```python
from build123d import *

# Parameters (mm, degrees)
SKETCH006_W     = 112.91
SKETCH006_H     = 87.54
SKETCH006_R     = 3
SKETCH006_R_2   = 2.65
SKETCH006_R_3   = 36
PAD005_DEPTH    = 1.6
CHAMFER_SIZE    = 1
SKETCH007_W     = 112.91
SKETCH007_H     = 87.54
SKETCH007_R     = 3
PAD006_DEPTH    = 1.8
SKETCH009_W     = 112.91
SKETCH009_H     = 87.54
SKETCH009_R     = 1.75
PAD007_DEPTH    = 28.2
SKETCH008_W     = 44
SKETCH008_H     = 25
POCKET_DEPTH    = 1.22
POCKET001_DEPTH = 1.22
SKETCH011_W     = 95.03
SKETCH011_H     = 22
POCKET002_DEPTH = 1.22
SKETCH012_W     = 42.2
SKETCH012_H     = 22
SKETCH012_W_2   = 15.44
SKETCH012_H_2   = 2
SKETCH012_W_3   = 12.5
SKETCH012_H_3   = 12
POCKET003_DEPTH = 1.22
FILLET001_R     = 1


with BuildPart() as part:
    # Sketch006 → Pad005 (new body)
    with BuildSketch(Plane.XY):
        Rectangle(SKETCH006_W, SKETCH006_H)
        with Locations((-50.925, 38.05)):
            Circle(SKETCH006_R, mode=Mode.SUBTRACT)
        with Locations((50.925, 38.05)):
            Circle(SKETCH006_R, mode=Mode.SUBTRACT)
        with Locations((-50.925, -38.05)):
            Circle(SKETCH006_R, mode=Mode.SUBTRACT)
        with Locations((50.925, -38.05)):
            Circle(SKETCH006_R, mode=Mode.SUBTRACT)
        with Locations((-43.265, 35.75)):
            Circle(SKETCH006_R_2, mode=Mode.SUBTRACT)
        with Locations((28.235, 35.75)):
            Circle(SKETCH006_R_2, mode=Mode.SUBTRACT)
        with Locations((28.235, -35.75)):
            Circle(SKETCH006_R_2, mode=Mode.SUBTRACT)
        with Locations((-43.265, -35.75)):
            Circle(SKETCH006_R_2, mode=Mode.SUBTRACT)
        with Locations((-7.515, 0)):
            Circle(SKETCH006_R_3, mode=Mode.SUBTRACT)
    extrude(amount=PAD005_DEPTH)

    # Chamfer
    chamfer_edges = [part.edges().sort_by_distance(p)[0] for p in [
        (-45.915, 35.75, 1.6),
        (25.585, 35.75, 1.6),
        (-45.915, -35.75, 1.6),
        (25.585, -35.75, 1.6),
    ]]
    chamfer(chamfer_edges, length=CHAMFER_SIZE)

    # Sketch007 → Pad006 (join)
    with BuildSketch(Plane.XY.offset(1.6)):
        Rectangle(SKETCH007_W, SKETCH007_H)
        with Locations((-50.925, 38.05)):
            Circle(SKETCH007_R, mode=Mode.SUBTRACT)
        with Locations((50.925, 38.05)):
            Circle(SKETCH007_R, mode=Mode.SUBTRACT)
        with Locations((-50.925, -38.05)):
            Circle(SKETCH007_R, mode=Mode.SUBTRACT)
        with Locations((50.925, -38.05)):
            Circle(SKETCH007_R, mode=Mode.SUBTRACT)
        with BuildLine():
            Line((-47.515, 42.55), (47.515, 42.55))
            Line((47.515, 42.55), (47.515, 38.05))
            ThreePointArc((47.515, 38.05), (48.513766, 35.638766), (50.925, 34.64))
            Line((55.235, 34.64), (50.925, 34.64))
            Line((55.235, -34.64), (55.235, 34.64))
            Line((55.235, -34.64), (50.925, -34.64))
            ThreePointArc((50.925, -34.64), (48.513766, -35.638766), (47.515, -38.05))
            Line((47.515, -42.55), (47.515, -38.05))
            Line((-47.515, -42.55), (47.515, -42.55))
            Line((-47.515, -42.55), (-47.515, -38.05))
            ThreePointArc((-47.515, -38.05), (-48.513766, -35.638766), (-50.925, -34.64))
            Line((-55.235, -34.64), (-50.925, -34.64))
            Line((-55.235, 34.64), (-55.235, -34.64))
            Line((-55.235, 34.64), (-50.925, 34.64))
            ThreePointArc((-50.925, 34.64), (-48.513766, 35.638766), (-47.515, 38.05))
            Line((-47.515, 42.55), (-47.515, 38.05))
        make_face(mode=Mode.SUBTRACT)
    extrude(amount=PAD006_DEPTH)

    # Sketch009 → Pad007 (join)
    with BuildSketch(Plane.XY.offset(3.4)):
        Rectangle(SKETCH009_W, SKETCH009_H)
        with Locations((-50.925, 38.05)):
            Circle(SKETCH009_R, mode=Mode.SUBTRACT)
        with Locations((50.925, 38.05)):
            Circle(SKETCH009_R, mode=Mode.SUBTRACT)
        with Locations((-50.925, -38.05)):
            Circle(SKETCH009_R, mode=Mode.SUBTRACT)
        with Locations((50.925, -38.05)):
            Circle(SKETCH009_R, mode=Mode.SUBTRACT)
        with BuildLine():
            Line((-47.515, 42.55), (47.515, 42.55))
            Line((47.515, 42.55), (47.515, 38.05))
            ThreePointArc((47.515, 38.05), (48.513766, 35.638766), (50.925, 34.64))
            Line((55.235, 34.64), (50.925, 34.64))
            Line((55.235, -34.64), (55.235, 34.64))
            Line((55.235, -34.64), (50.925, -34.64))
            ThreePointArc((50.925, -34.64), (48.513766, -35.638766), (47.515, -38.05))
            Line((47.515, -42.55), (47.515, -38.05))
            Line((-47.515, -42.55), (47.515, -42.55))
            Line((-47.515, -42.55), (-47.515, -38.05))
            ThreePointArc((-47.515, -38.05), (-48.513766, -35.638766), (-50.925, -34.64))
            Line((-55.235, -34.64), (-50.925, -34.64))
            Line((-55.235, 34.64), (-55.235, -34.64))
            Line((-55.235, 34.64), (-50.925, 34.64))
            ThreePointArc((-50.925, 34.64), (-48.513766, 35.638766), (-47.515, 38.05))
            Line((-47.515, 42.55), (-47.515, 38.05))
        make_face(mode=Mode.SUBTRACT)
    extrude(amount=PAD007_DEPTH)

    # Sketch008 → Pocket (cut)
    with BuildSketch(Plane(origin=(56.455, 0, 1.6), x_dir=(0, 1, 0), z_dir=(1, 0, 0))):
        with Locations((1.85, 17.5)):
            Rectangle(SKETCH008_W, SKETCH008_H)
    extrude(amount=-POCKET_DEPTH, mode=Mode.SUBTRACT)

    # Sketch010 → Pocket001 (cut)
    with BuildSketch(Plane(origin=(-56.455, 0, 1.6), x_dir=(0, -1, 0), z_dir=(-1, 0, 0))):
        Polygon((-34.65, 30), (18.85, 30), (18.85, 12), (10.85, 12), (10.85, 20), (-34.65, 20), align=None)
    extrude(amount=-POCKET001_DEPTH, mode=Mode.SUBTRACT)

    # Sketch011 → Pocket002 (cut)
    with BuildSketch(Plane(origin=(0, -43.77, 1.6), x_dir=(1, 0, 0), z_dir=(0, -1, 0))):
        with Locations((0, 19)):
            Rectangle(SKETCH011_W, SKETCH011_H)
    extrude(amount=-POCKET002_DEPTH, mode=Mode.SUBTRACT)

    # Sketch012 → Pocket003 (cut)
    with BuildSketch(Plane(origin=(0, 43.77, 1.6), x_dir=(-1, 0, 0), z_dir=(0, 1, 0))):
        with Locations((-25.735, 19)):
            Rectangle(SKETCH012_W, SKETCH012_H)
        with Locations((4.855, 29)):
            Rectangle(SKETCH012_W_2, SKETCH012_H_2)
        with Locations((24.785, 24)):
            Rectangle(SKETCH012_W_3, SKETCH012_H_3)
    extrude(amount=-POCKET003_DEPTH, mode=Mode.SUBTRACT)

    # Fillet001
    fillet001_edges = [part.edges().sort_by_distance(p)[0] for p in [
        (56.455, -43.77, 15.8),
        (56.455, 0, 0),
        (0, -43.77, 0),
        (56.455, 43.77, 15.8),
        (0, 43.77, 0),
        (-56.455, 0, 0),
        (-56.455, -43.77, 15.8),
        (-56.455, 43.77, 15.8),
        (-48.513766, -35.638766, 1.6),
        (-55.235, 0, 1.6),
        (0, -42.55, 1.6),
        (-48.513766, 35.638766, 1.6),
        (48.513766, -35.638766, 1.6),
        (0, 42.55, 1.6),
        (48.513766, 35.638766, 1.6),
        (55.235, 0, 1.6),
    ]]
    fillet(fillet001_edges, radius=FILLET001_R)


solid = part.part
```
Model file for the job. Use its own axes, mm. A direction names the side the tool comes from. Round coordinates to 2 decimals unless told otherwise and drop trailing zeros. Order: outer loops, then holes, each group sorted by start corner. A loop starts at its lowest first (then second) coordinate and runs counter-clockwise, first axis right, second up. Notation, with made-up numbers: M -23,-25.5 L 24,-25.5 A19 ccw 24,-10.5 Z; hole C 70,73 d10. An arc over 180 degrees is marked long. Use CSV: the item, a comma, the result in double quotes.
Item 1: Which spindle directions (+Z, -Z, +X, -X, +Y, -Y) get a long thin tool onto all of the face, cutting with end or side? Do faces 4 (the face through (53, 34.64, 17)), 5 (the face through (-49, 38, 3.4)), 6 (the face through (49.635, 39.233, 17.303)). Say none if no direction does.
Worked answers:
face 4,"+Z"
face 5,"-Z"
face 6,"+Z, -Z"
Item 2: Saw through at D-D (x = -16.5). List the corners of the cut face in (y, z).
Worked answers:
outline,"M -43.77,1 A1 ccw -42.77,0 L -34.86,0 L -34.86,1.6 L -41.55,1.6 A1 cw -42.55,2.6 L -42.55,9.6 L -43.77,9.6 Z; M 34.86,0 L 42.77,0 A1 ccw 43.77,1 L 43.77,31.6 L 42.55,31.6 L 42.55,2.6 A1 cw 41.55,1.6 L 34.86,1.6 Z"
Item 3: Saw through at C-C (z = 17). State how many separate pieces and enclosed holes the cut face has, plus the area to 3 significant figures.
Worked answers:
separate pieces,"4"
enclosed holes,"4"
area,"447 mm²"
Item 4: Saw through at A-A (y = 0). List the corners of the cut face in (x, z) (3 decimals), plus the area to 3 significant figures.
Worked answers:
outline,"M -56.455,1 A1 ccw -55.455,0 L -43.515,0 L -43.515,1.6 L -54.235,1.6 A1 cw -55.235,2.6 L -55.235,21.6 L -56.455,21.6 Z; M 28.485,0 L 55.455,0 A1 ccw 56.455,1 L 56.455,6.6 L 55.235,6.6 L 55.235,2.6 A1 cw 54.235,1.6 L 28.485,1.6 Z"
area,"96.0 mm²"
Item 5: Probe probe 1 along X at (y, z) = (38, 23) (3 decimals); probe 2 along Y at (x, z) = (-1, 3); probe 3 along X at (y, z) = (32, 5.5) (3 decimals). List the from-to ranges inside material, lowest first.
Worked answers:
probe 1,"-56.455 to -52.674, -49.176 to -47.515, 47.515 to 49.176, 52.674 to 56.455"
probe 2,"-43.77 to -42.55, 42.55 to 43.77"
probe 3,"-56.455 to -55.235, 55.235 to 56.455"
Item 6: Pull direction X, two halves, no side cores. Call faces 1 (the face through (-49, 41, 31.6)), 2 (the face through (-56.455, -1, 13)), 3 (the face through (-11, 42.55, 14)): released by +X, released by -X, zero draft, split by the parting line, or undercut.
Worked answers:
face 1,"zero draft"
face 2,"released by -X"
face 3,"undercut"
Item 7: Pin check, flat tips, straight feed: pin 1 (0.6 mm diameter, centred on x = -56, y = -16, fed in from +Z); pin 2 (1.5 mm diameter, centred on x = 39, y = -32.5, fed in from +Z); pin 3 (6 mm diameter, centred on x = 7.5, z = 24.5, fed in from -Y); pin 4 (8 mm diameter, centred on y = -9.5, z = 28, fed in from +X). Stop position of each tip, or through.
Worked answers:
pin 1,"z = 13.6"
pin 2,"z = 1.6"
pin 3,"y = 42.55"
pin 4,"through"
Item 8: Saw through at B-B (z = 5). List the corners of the cut face in (x, y) (3 decimals), plus the area to 3 significant figures.
Worked answers:
outline,"M -56.455,-42.77 A1 ccw -55.455,-43.77 L 55.455,-43.77 A1 ccw 56.455,-42.77 L 56.455,42.77 A1 ccw 55.455,43.77 L -55.455,43.77 A1 ccw -56.455,42.77 Z; hole M -55.235,-34.64 L -50.925,-34.64 A3.41 cw -47.515,-38.05 L -47.515,-42.55 L 47.515,-42.55 L 47.515,-38.05 A3.41 cw 50.925,-34.64 L 55.235,-34.64 L 55.235,34.64 L 50.925,34.64 A3.41 cw 47.515,38.05 L 47.515,42.55 L -47.515,42.55 L -47.515,38.05 A3.41 cw -50.925,34.64 L -55.235,34.64 Z; hole C -50.925,-38.05 d3.5; hole C -50.925,38.05 d3.5; hole C 50.925,-38.05 d3.5; hole C 50.925,38.05 d3.5"
area,"678 mm²"
